Could you check a few things on this model? Use its own coordinates, in mm. A direction names the side the tool comes from. Round coordinates to 2 decimals unless told otherwise and drop trailing zeros. Loops run counter-clockwise (first coordinate to the right, second up) from the corner with the lowest first, then second, coordinate; pieces in that order, holes last. Notation, with made-up numbers: (-16, 16) - (23, 16) arc R14 cw to (23, 40) - close; hole circle Ø3 at (23, -31.5). An arc over 180 degrees is marked (long way). Use one line per item in the form item = value.
```python
from build123d import *

# Parameters (mm, degrees)
SKETCH2_R           = 50.8
BOSS_EXTRUDE1_DEPTH = 4.064
SKETCH3_W           = 87.988181024
SKETCH3_H           = 5.08
BOSS_EXTRUDE2_DEPTH = 50.8
CUT_EXTRUDE2_DEPTH  = 77.2
FILLET1_R           = 36.322
SKETCH6_R           = 15.24
CUT_EXTRUDE3_DEPTH  = 77.2
SKETCH7_R           = 3.175
CUT_EXTRUDE4_DEPTH  = 5.064


with BuildPart() as part:
    # Sketch2 → Boss-Extrude1 (new body)
    with BuildSketch(Plane(origin=(0, 0, 0), x_dir=(1, 0, 0), z_dir=(0, 1, 0))):
        Circle(SKETCH2_R)
    extrude(amount=BOSS_EXTRUDE1_DEPTH)

    # Sketch3 → Boss-Extrude2 (add)
    with BuildSketch(Plane(origin=(0, 4.064, 0), x_dir=(1, 0, 0), z_dir=(0, 1, 0))):
        with Locations((0, -22.86)):
            Rectangle(SKETCH3_W, SKETCH3_H)
        with Locations((0, 22.86)):
            Rectangle(SKETCH3_W, SKETCH3_H)
    extrude(amount=BOSS_EXTRUDE2_DEPTH)

    # Sketch5 → Cut-Extrude2 (cut, through all)
    with BuildSketch(Plane(origin=(0, 0, -25.4), x_dir=(-1, 0, 0), z_dir=(0, 0, -1))):
        Polygon((-43.994090512, 4.064), (-43.994090512, 54.864), (-36.374090512, 54.864), align=None)
        Polygon((43.994090512, 4.064), (36.374090512, 54.864), (43.994090512, 54.864), align=None)
    extrude(amount=-CUT_EXTRUDE2_DEPTH, mode=Mode.SUBTRACT)

    # Fillet1
    fillet1_edges = [part.edges().sort_by_distance(p)[0] for p in [
        (36.374090512, 54.864, -22.86),
        (36.374090512, 54.864, 22.86),
        (-36.374090512, 54.864, -22.86),
        (-36.374090512, 54.864, 22.86),
    ]]
    fillet(fillet1_edges, radius=FILLET1_R)

    # Sketch6 → Cut-Extrude3 (cut, through all)
    with BuildSketch(Plane(origin=(0, 0, -25.4), x_dir=(-1, 0, 0), z_dir=(0, 0, -1))):
        with Locations((0, 29.464)):
            Circle(SKETCH6_R)
    extrude(amount=-CUT_EXTRUDE3_DEPTH, mode=Mode.SUBTRACT)

    # Sketch7 → Cut-Extrude4 (cut, through all)
    with BuildSketch(Plane(origin=(0, 4.064, 0), x_dir=(1, 0, 0), z_dir=(0, 1, 0))):
        Circle(SKETCH7_R)
    extrude(amount=-CUT_EXTRUDE4_DEPTH, mode=Mode.SUBTRACT)


solid = part.part
```
1. For P1, Ø10, axis at y = 10.5, z = -33.5, coming from the -X side; P2, Ø15, axis at x = -18, y = 41, coming from the -Z side; P3, Ø6, axis at x = 6, y = 12.5, coming from the +Z side; P4, Ø2, axis at x = -28.5, z = -26.5, coming from the -Y side, each with a flat end and sliding along its axis, tell me the tip position at first contact or that it passes through.
Solution:
P1 = through
P2 = -25.4
P3 = 25.4
P4 = 0
2. If we section it at B-B, the plane x = 0: Write out the boundary of the cut face in (y, z) (3 decimals), plus the area to 3 significant figures.
Solution:
outline = (0, -50.8) - (4.064, -50.8) - (4.064, -25.4) - (14.224, -25.4) - (14.224, -20.32) - (4.064, -20.32) - (4.064, -3.175) - (0, -3.175) - close; (0, 3.175) - (4.064, 3.175) - (4.064, 20.32) - (14.224, 20.32) - (14.224, 25.4) - (4.064, 25.4) - (4.064, 50.8) - (0, 50.8) - close; (44.704, -25.4) - (54.864, -25.4) - (54.864, -20.32) - (44.704, -20.32) - close; (44.704, 20.32) - (54.864, 20.32) - (54.864, 25.4) - (44.704, 25.4) - close
area = 594 mm^2
3. On a 3-axis mill with a long thin cutter (end or side, diameter ignored), from which of +Z, -Z, +X, -X, +Y, -Y can I reach the whole of each face in a straight line? I mean faces 1 (the face through (0, 54.864, -23)), 2 (the face through (-10.4, 17.8, -25.4)), 3 (the face through (42.483, 14.136, 22.824)), 4 (the face through (-1, 4.064, 35)), 5 (the face through (-10.4, 17.8, -20.32)). Say none if no direction works.
Solution:
face_1 = +Z, -Z, +X, -X, +Y
face_2 = -Z, +X, -X, +Y
face_3 = +Z, -Z, +X, +Y
face_4 = +Z, +X, -X, +Y
face_5 = +X, -X, +Y
4. If we section it at C-C, the plane y = 11.5: Write out the boundary of the cut face in (x, z).
Solution:
outline = (-42.88, -25.4) - (42.88, -25.4) - (42.88, -20.32) - (-42.88, -20.32) - close; (-42.88, 20.32) - (42.88, 20.32) - (42.88, 25.4) - (-42.88, 25.4) - close
5. We'd pull the mould along Z, two halves only. Please class faces 6 (the face through (-11.012, 2.004, 49.592)), 7 (the face through (29.1, 45.8, -22.8)), 8 (the face through (-1, 4.064, -6)): +Z half, -Z half, draft (parallel to the pull), parting line (faces both ways), or undercut.
Solution:
face_6 = parting line
face_7 = draft
face_8 = undercut
6. If we section it at A-A, the plane z = 0: Write out the boundary of the cut face in (x, y) (3 decimals), plus the area to 3 significant figures.
Solution:
outline = (-50.8, 0) - (-3.175, 0) - (-3.175, 4.064) - (-50.8, 4.064) - close; (3.175, 0) - (50.8, 0) - (50.8, 4.064) - (3.175, 4.064) - close
area = 387 mm^2
7. If we section it at D-D, the plane y = 17.5: Write out the boundary of the cut face in (x, z), plus the area to 3 significant figures.
Solution:
outline = (-41.98, -25.4) - (-9.44, -25.4) - (-9.44, -20.32) - (-41.98, -20.32) - close; (-41.98, 20.32) - (-9.44, 20.32) - (-9.44, 25.4) - (-41.98, 25.4) - close; (9.44, -25.4) - (41.98, -25.4) - (41.98, -20.32) - (9.44, -20.32) - close; (9.44, 20.32) - (41.98, 20.32) - (41.98, 25.4) - (9.44, 25.4) - close
area = 661 mm^2
8. Please list where these lines run through material, in increasing order: line 1 along X through (y, z) = (1, 0) (3 decimals); line 2 along Z through (x, y) = (16, 37); line 3 along Y through (x, z) = (0, -23).
Solution:
line_1 = -50.8 to -3.175, 3.175 to 50.8
line_2 = -25.4 to -20.32, 20.32 to 25.4
line_3 = 0 to 14.22, 44.7 to 54.86
